The listing builds one solid part. Answer for the finished solid, in the listing's coordinates (mm). A direction names the side the tool comes from. Coordinates: 2 decimals unless noted, no trailing zeros. Loops run counter-clockwise (first coordinate to the right, second up) from the corner with the lowest first, then second, coordinate; pieces in that order, holes last. Notation, with made-up numbers: (-28, 12) - (-3, 12) arc R10 ccw to (-3, 31) - close; hole circle Ø5 at (43, 57). An arc over 180 degrees is marked (long way). Use one line per item in the form item = value. Start each with the question number.
```python
from build123d import *

# Parameters (mm, degrees)
F0_W      = 914.4
F0_H      = 609.6
F1_DEPTH  = 25.4
F2_SIZE   = 127
F3_W      = 609.6
F3_H      = 203.2
F4_DEPTH  = 25.4
F5_W      = 660.4
F5_H      = 254
F5_W_2    = 609.6
F5_H_2    = 203.2
F6_DEPTH  = 127
F7_W      = 660.4
F7_H      = 254
F8_DEPTH  = 25.4
F9_W      = 635
F9_H      = 228.6
F10_DEPTH = 12.7


with BuildPart() as f1:
    # F0 (on Top) → F1 (new body)
    with BuildSketch(Plane.XY):
        Rectangle(F0_W, F0_H)
    extrude(amount=F1_DEPTH)

    # F2
    f2_edges = [f1.edges().sort_by_distance(p)[0] for p in [
        (-457.2, -304.8, 12.7),
        (457.2, -304.8, 12.7),
        (457.2, 304.8, 12.7),
        (-457.2, 304.8, 12.7),
    ]]
    chamfer(f2_edges, length=F2_SIZE)

    # F3 (on face) → F4 (cut, through all)
    with BuildSketch(Plane.XY.offset(25.4)):
        Rectangle(F3_W, F3_H)
    extrude(amount=-F4_DEPTH, mode=Mode.SUBTRACT)

    # F5 (on face) → F6 (join)
    with BuildSketch(Plane(origin=(0, 0, 0), x_dir=(1, 0, 0), z_dir=(0, 0, -1))):
        Rectangle(F5_W, F5_H)
        Rectangle(F5_W_2, F5_H_2, mode=Mode.SUBTRACT)
    extrude(amount=F6_DEPTH)

    # F7 (on face) → F8 (join)
    with BuildSketch(Plane(origin=(0, 0, -127), x_dir=(1, 0, 0), z_dir=(0, 0, -1))):
        Rectangle(F7_W, F7_H)
    extrude(amount=F8_DEPTH)

    # F9 (on face) → F10 (cut)
    with BuildSketch(Plane.XY.offset(25.4)):
        Rectangle(F9_W, F9_H)
    extrude(amount=-F10_DEPTH, mode=Mode.SUBTRACT)


solid = f1.part
```
(1) A cutting plane is placed at B-B (x = -54.5). Determine the outline of the cut face in (y, z).
(2) Find the intervals of material crossed by probe 1 along Y at (x, z) = (-305, 16.5); probe 2 along Y at (x, z) = (-145, -15.5); probe 3 along X at (y, z) = (-88.5, -90), in increasing order. Write a range as from..to.
(3) Determine the mould class of faces 6 (the face through (-304.8, 1, -56)), 7 (the face through (-393, 242, 13)), 8 (the face through (457.2, -2, 13)), 9 (the face through (-96, 102, 12.7)) for opening direction Y: +Y half, -Y half, draft (parallel to the pull), parting line (faces both ways), or undercut.
(4) A cutting plane is placed at D-D (z = -137.5). Determine the outline of the cut face in (x, y).
(5) For faces 1 (the face through (-393, -242, 13)), 2 (the face through (-330.2, 2, -75)), 3 (the face through (-4, 101.6, -56)), 4 (the face through (330.2, 2, -75)), 5 (the face through (-5, -127, -75)), determine the directions among +Z, -Z, +X, -X, +Y, -Y from which every point of the face is accessible in a straight line to the end or side of a thin tool.
(6) A cutting plane is placed at A-A (z = -98). Determine the outline of the cut face in (x, y), then the cut area to 3 significant figures.
(7) A cutting plane is placed at C-C (y = -30). Determine the outline of the cut face in (x, z).
(8) Each of these flat-tipped pins is pushed along its axis until it touches: pin 1 Ø10 at (y, z) = (59, -77) entering from +X; pin 2 Ø4 at (x, z) = (-162.5, -15) entering from -Y; pin 3 Ø6 at (x, z) = (130.5, -71) entering from +Y. Where does it stop, or does it pass through?
Evaluation:
q1.outline = (-304.8, 0) - (-127, 0) - (-127, -152.4) - (127, -152.4) - (127, 0) - (304.8, 0) - (304.8, 25.4) - (114.3, 25.4) - (114.3, 12.7) - (101.6, 12.7) - (101.6, -127) - (-101.6, -127) - (-101.6, 12.7) - (-114.3, 12.7) - (-114.3, 25.4) - (-304.8, 25.4) - close
q2.probe_1 = -304.8..-114.3, 114.3..304.8
q2.probe_2 = -127..-101.6, 101.6..127
q2.probe_3 = -330.2..-304.8, 304.8..330.2
q3.face_6 = undercut
q3.face_7 = +Y half
q3.face_8 = draft
q3.face_9 = undercut
q4.outline = (-330.2, -127) - (330.2, -127) - (330.2, 127) - (-330.2, 127) - close
q5.face_1 = +Z, -Z, -X, -Y
q5.face_2 = -Z, -X, +Y, -Y
q5.face_3 = +Z
q5.face_4 = -Z, +X, +Y, -Y
q5.face_5 = -Z, +X, -X, -Y
q6.outline = (-330.2, -127) - (330.2, -127) - (330.2, 127) - (-330.2, 127) - close; hole (-304.8, -101.6) - (304.8, -101.6) - (304.8, 101.6) - (-304.8, 101.6) - close
q6.area = 43,900 mm^2
q7.outline = (-457.2, 0) - (-330.2, 0) - (-330.2, -152.4) - (330.2, -152.4) - (330.2, 0) - (457.2, 0) - (457.2, 25.4) - (317.5, 25.4) - (317.5, 12.7) - (304.8, 12.7) - (304.8, -127) - (-304.8, -127) - (-304.8, 12.7) - (-317.5, 12.7) - (-317.5, 25.4) - (-457.2, 25.4) - close
q8.pin_1 = 330.2
q8.pin_2 = -127
q8.pin_3 = 127
